Answer from the drawing. Dimensions are ordinates in mm from the lowest x, y and z of the part. Give positions to 0.01 mm unless a question says otherwise; leave off trailing zeros. Write each loop counter-clockwise with the first axis right and the second up, starting at its lowest first coordinate (ties: lowest second). Pieces come first, ordered by that corner, then holes. Notation, with made-up numbers: M 80.5,5 L 88.5,5 A29 ccw 88.5,42 Z; hole C 30.5,-26.75 d10. An arc over 180 degrees is marked long. Put each result on its own line as item: value.
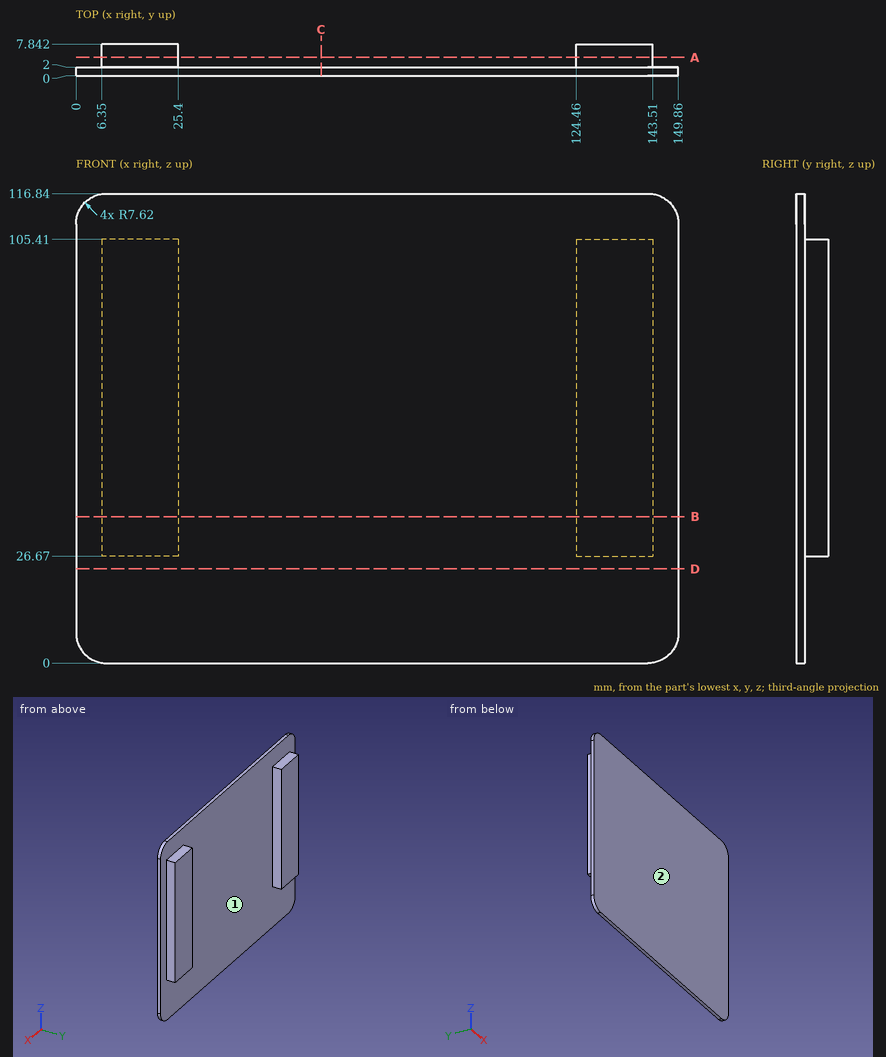
(1) For a pull along X with two mould halves and no side action, classify the marked faces 1 and 2 as +X half, -X half, draft (parallel to the pull), parting line (faces both ways), or undercut.
Result:
face 1: undercut
face 2: draft
(2) Straight lines are drawn through the part: line 1 along X through (y, z) = (4.25, 75); line 2 along Z through (x, y) = (135, 3.25); line 3 along Y through (x, z) = (37.5, 54.5). For each, find the intervals that lie inside material, in ascending order. Write a range as from..to.
Result:
line 1: x = 6.35..25.4, 124.46..143.51
line 2: z = 26.67..105.41
line 3: y = 0..2
(3) Section B-B on z = 36.5 is taken. Determine the outline of the cut face in (x, y).
Result:
outline: M 0,0 L 149.86,0 L 149.86,2 L 143.51,2 L 143.51,7.84 L 124.46,7.84 L 124.46,2 L 25.4,2 L 25.4,7.84 L 6.35,7.84 L 6.35,2 L 0,2 Z
(4) Section D-D on z = 23.5 is taken. Determine the outline of the cut face in (x, y), and give its area (3 significant figures).
Result:
outline: M 0,0 L 149.86,0 L 149.86,2 L 0,2 Z
area: 300 mm²
(5) Given pin 1 Ø4.5 at (x, y) = (17.5, 5.5) entering from -Z; pin 2 Ø3 at (y, z) = (4, 69) entering from +X; pin 3 Ø3 at (x, y) = (16, 6) entering from +Z, each flat-ended and moving along its own axis, determine where each tip first touches the part or whether it passes through.
Result:
pin 1: stops at z = 26.67
pin 2: stops at x = 143.51
pin 3: stops at z = 105.41
(6) Section C-C on x = 61 is taken. Determine the outline of the cut face in (y, z).
Result:
outline: M 0,0 L 2,0 L 2,116.84 L 0,116.84 Z
(7) Section A-A on y = 4.5 is taken. Determine the outline of the cut face in (x, z).
Result:
outline: M 6.35,26.67 L 25.4,26.67 L 25.4,105.41 L 6.35,105.41 Z; M 124.46,26.67 L 143.51,26.67 L 143.51,105.41 L 124.46,105.41 Z
